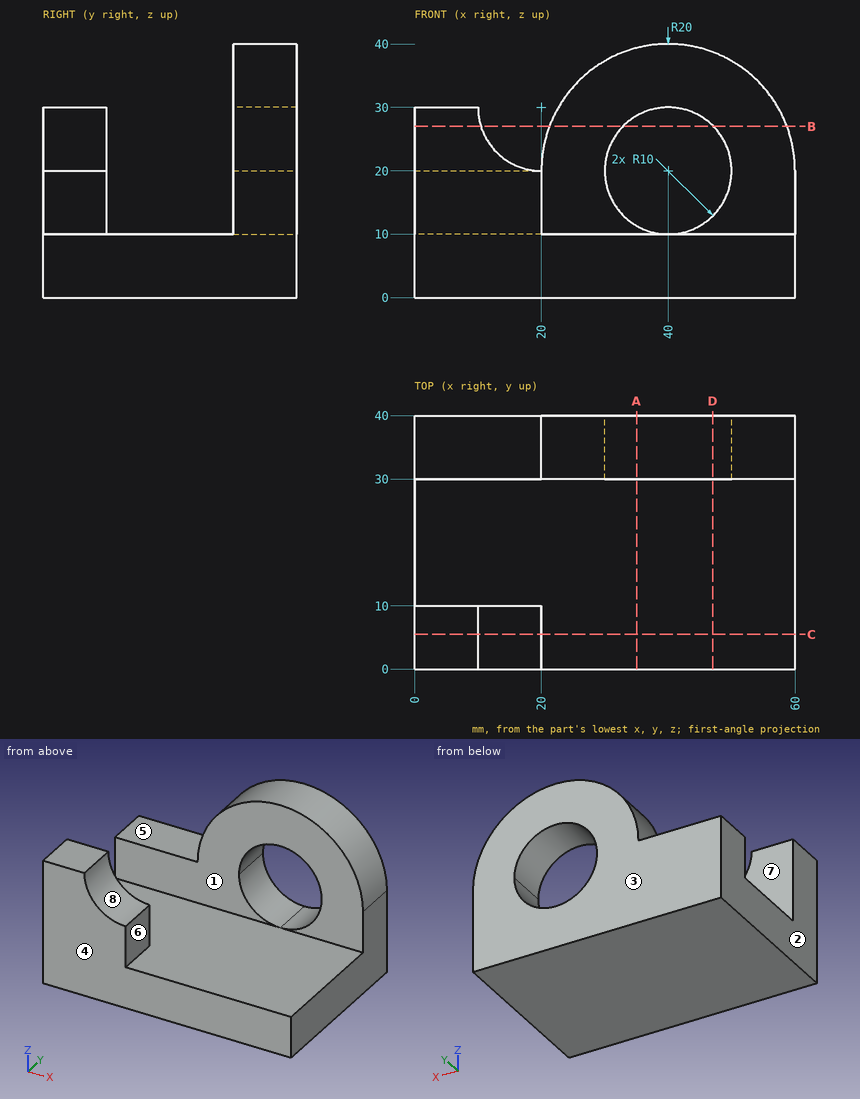
Print and shaded views of the part. All mm, measured from the part's lowest x, y and z. A direction names the side the tool comes from. Give positions to 0.01 mm unless a question says otherwise; leave off trailing zeros. Write each loop counter-clockwise with the first axis right and the second up, starting at its lowest first coordinate (ties: lowest second). Pieces come first, ordered by that corner, then holes. Notation, with made-up numbers: (45.25, 26.25) - (78.25, 26.25) arc R15 ccw to (78.25, 32.25) - close; hole circle Ø9 at (40, 34). An arc over 180 degrees is marked (long way). One line per question, with ' | ' between items. Start each with the question number.
(1) Slice it at C-C on y = 5.5. Write the cut outline in (x, z).
(2) Pin check, flat tips, straight feed: P1, Ø1, axis at y = 30.5, z = 36, coming from the -X side; P2, Ø24, axis at x = 35, y = 17.5, coming from the +Z side; P3, Ø8, axis at y = 7.5, z = 17, coming from the +X side. Stop position of each tip, or through.
(3) Slice it at A-A on x = 35. Write the cut outline in (y, z), plus the area to 3 significant figures.
(4) Wall check: line 1 along Y through (x, z) = (16, 13.5); line 2 along Z through (x, y) = (18, 21); line 3 along X through (y, z) = (31, 19.5). Give the ranges that are in metal, low to high. Write a range as from..to.
(5) Slice it at D-D on x = 47. Write the cut outline in (y, z) (3 decimals).
(6) 3-axis set-ups, long thin cutter, end or side, ignore diameter. For the marked faces 5, 6, 7 and 8: which of +Z, -Z, +X, -X, +Y, -Y reach the whole face in a straight line?
(7) Slice it at B-B on z = 27. Write the cut outline in (x, y) (3 decimals).
(8) Two-plate mould, pull along Y, no slides. Class the marked faces 1, 2, 3 and 4: +Y half, -Y half, draft (parallel to the pull), parting line (faces both ways), or undercut.
Results below:
1) outline: (0, 0) - (60, 0) - (60, 10) - (20, 10) - (20, 20) arc R10 cw to (10, 30) - (0, 30) - close
2) P1: x = 27.36 | P2: z = 10 | P3: x = 20
3) outline: (0, 0) - (40, 0) - (40, 11.34) - (30, 11.34) - (30, 10) - (0, 10) - close; (30, 28.66) - (40, 28.66) - (40, 39.36) - (30, 39.36) - close | area: 520 mm^2
4) line 1: 0..10, 30..40 | line 2: 0..10 | line 3: 0..30.01, 49.99..60
5) outline: (0, 0) - (40, 0) - (40, 12.859) - (30, 12.859) - (30, 10) - (0, 10) - close; (30, 27.141) - (40, 27.141) - (40, 38.735) - (30, 38.735) - close
6) face 5: +Z, -X, +Y | face 6: +Z, +X, -Y | face 7: +Z, +X, -X | face 8: +Z, +X, +Y, -Y
7) outline: (0, 0) - (10.461, 0) - (10.461, 10) - (0, 10) - close; (21.265, 30) - (32.859, 30) - (32.859, 40) - (21.265, 40) - close; (47.141, 30) - (58.735, 30) - (58.735, 40) - (47.141, 40) - close
8) face 1: undercut | face 2: draft | face 3: +Y half | face 4: -Y half
